Design review of the part built by this model. Coordinates are the model's own, in mm. A direction names the side the tool comes from. Give positions to 0.01 mm unless a question says otherwise; leave off trailing zeros. Order: outer loops, then holes, each group sorted by start corner. A loop starts at its lowest first (then second) coordinate and runs counter-clockwise, first axis right, second up. Notation, with made-up numbers: M -4,47.25 L 44,47.25 A34 ccw 44,77.25 Z; hole C 79,0 d5. An arc over 180 degrees is marked long. Answer as a JSON object with one key per item and string values.
Autodesk Inventor part; units mm, degrees
ref_plane "YZ Plane" through (0, 0, 0) normal (1, 0, 0) x (0, 1, 0)
ref_plane "XZ Plane" through (0, 0, 0) normal (0, 1, 0) x (-1, 0, 0)
ref_plane "XY Plane" through (0, 0, 0) normal (0, 0, 1) x (1, 0, 0)
sketch "Sketch1" plane through (0, 0, 0) normal (0, 1, 0) x (-1, 0, 0)
  line L0 (0, 0) -> (-361.95, 0)
  line L1 (-361.95, 0) -> (-361.95, -463.55)
  line L2 (-361.95, -463.55) -> (0, -463.55)
  line L3 (0, -463.55) -> (0, 0)
  dimension "d0" = 361.95
  dimension "d1" = 463.55
extrude "Extrusion1" add sketch "Sketch1" along normal blind 2.794
fillet "Fillet1" radius 19.05 4 edges at (361.95, 1.397, 0) (361.95, 1.397, -463.55) (0, 1.397, -463.55) (0, 1.397, 0)
sketch "Sketch2" plane through (0, 0, 0) normal (0, -1, 0) x (1, 0, 0)
  line L0 (19.05, 0) -> (342.9, 0)
  line L1 (342.9, 0) -> (342.9, -2.8525)
  line L2 (342.9, -2.8525) -> (19.05, -2.8525)
  line L3 (19.05, -2.8525) -> (19.05, 0)
  line L4 (342.9, -2.8525) -> (317.5, -2.8525)
  line L5 (317.5, -2.8525) -> (317.5, 0)
  line L6 (317.5, 0) -> (342.9, 0)
  line L7 (342.9, 0) -> (342.9, -2.8525)
  line L8 (19.05, -2.8525) -> (44.45, -2.8525)
  line L9 (44.45, -2.8525) -> (44.45, 0)
  line L10 (44.45, 0) -> (19.05, 0)
  line L11 (19.05, 0) -> (19.05, -2.8525)
  line L12 (44.45, -2.8525) -> (317.5, -2.8525)
  line L13 (317.5, -2.8525) -> (317.5, 0)
  line L14 (317.5, 0) -> (44.45, 0)
  line L15 (44.45, 0) -> (44.45, -2.8525)
  point P0 (0, 0)
  dimension "d5" = 25.4
  dimension "d6" = 25.4
extrude "Extrusion2" add sketch "Sketch2" along normal blind 25.4 contours L0 L5 L2 L9
sketch "Sketch3" plane through (19.05, 2.794, 0) normal (0, 0, 1) x (1, 0, 0)
  line L0 (323.85, -2.794) -> (0, -2.794)
  line L1 (25.405, -2.794) -> (25.4, -15.494)
  line L2 (25.4, -2.794) -> (25.4, -28.194)
  line L3 (25.4, -15.494) -> (85.4, -15.5178)
  line L4 (298.45, -2.794) -> (298.45, -28.194)
  line L5 (298.45, -15.494) -> (238.45, -15.494)
  circle A0 centre (85.4, -15.5178) radius 3.429
  circle A1 centre (238.45, -15.494) radius 3.429
  point P0 (-19.05, -2.794)
  dimension "d9" = 12.7
  dimension "d10" = 60
  dimension "d11" = 60
  dimension "d12" = 6.858
  dimension "d13" = 6.858
extrude "Extrusion3" cut sketch "Sketch3" against normal blind 25.4 contours A0 | A1
sketch "Sketch4" plane through (0, 2.794, 0) normal (0, 1, 0) x (1, 0, 0)
  arc A0 (0, 19.05) -> (19.05, 0) centre (19.05, 19.05) ccw
  line L0 (19.05, 0) -> (342.9, 0)
  arc A1 (342.9, 0) -> (361.95, 19.05) centre (342.9, 19.05) ccw
  line L1 (361.95, 19.05) -> (361.95, 444.5)
  arc A2 (361.95, 444.5) -> (342.9, 463.55) centre (342.9, 444.5) ccw
  line L2 (342.9, 463.55) -> (19.05, 463.55)
  arc A3 (19.05, 463.55) -> (0, 444.5) centre (19.05, 444.5) ccw
  line L3 (0, 444.5) -> (0, 19.05)
  point P0 (0, 0)
sketch "Sketch5" plane through (0, 2.794, 0) normal (0, 1, 0) x (1, 0, 0)
  arc A0 (0, 19.05) -> (19.05, 0) centre (19.05, 19.05) ccw
  line L0 (19.05, 0) -> (342.9, 0)
  arc A1 (342.9, 0) -> (361.95, 19.05) centre (342.9, 19.05) ccw
  line L1 (361.95, 19.05) -> (361.95, 444.5)
  arc A2 (361.95, 444.5) -> (342.9, 463.55) centre (342.9, 444.5) ccw
  line L2 (342.9, 463.55) -> (19.05, 463.55)
  arc A3 (19.05, 463.55) -> (0, 444.5) centre (19.05, 444.5) ccw
  line L3 (0, 444.5) -> (0, 19.05)
  line L4 (342.9, 444.5) -> (19.05, 19.05)
  line L5 (342.9, 19.05) -> (19.05, 444.5)
  line L6 (298.45, 425.45) -> (63.5, 425.45)
  line L7 (63.5, 425.45) -> (63.5, 38.1)
  line L8 (63.5, 38.1) -> (298.45, 38.1)
  line L9 (298.45, 38.1) -> (298.45, 425.45)
  line L10 (298.45, 425.45) -> (63.5, 38.1) construction
  line L11 (63.5, 425.45) -> (298.45, 38.1) construction
  point P0 (0, 0)
  point P1 (180.975, 231.775)
  dimension "d16" = 234.95
  dimension "d17" = 387.35
extrude "Extrusion4" cut sketch "Sketch5" against normal blind 25.4 contours L9 L5 L4 | L4 L5 L7 L6 L9 | L5 L9 L8 L7 L4 | L4 L7 L5
properties part number "Cart_TOP_SHELF" material "Cart Material"
(1) We need section C-C (y = -5). Write out the cut boundary in (x, z).
Checked values:
{"outline": "M 44.45,-2.85 L 317.5,-2.85 L 317.5,0 L 44.45,0 Z"}
(2) We need section A-A (z = -154). Write out the cut boundary in (x, y).
Checked values:
{"outline": "M 0,0 L 63.5,0 L 63.5,2.79 L 0,2.79 Z; M 298.45,0 L 361.95,0 L 361.95,2.79 L 298.45,2.79 Z"}
(3) Insertion check: pin 1 (0.9 mm diameter, centred on y = -19, z = -1.5, fed in from +X); pin 2 (2 mm diameter, centred on x = 287.5, y = -12, fed in from -Z); pin 3 (0.9 mm diameter, centred on y = -10, z = -1, fed in from -X). Each pin has a flat end and moves straight along its axis. Give the tip position at first contact, or say it passes through.
Checked values:
{"pin 1": "stops at x = 317.5", "pin 2": "stops at z = -2.85", "pin 3": "stops at x = 44.45"}
(4) Tool access review of faces 1 (the cylindrical face through (5.43, 1.42, -5.73)), 2 (the flat face through (183, -13, -2.852)): name each direction out of +Z, -Z, +X, -X, +Y, -Y from which nothing blocks a thin tool from reaching the whole face with its end or side.
Checked values:
{"face 1": "+Z, -X, +Y, -Y", "face 2": "-Z, +X, -X, -Y"}
(5) To check wall thickness, follow L1, parallel to Y at x = 104.45, z = -0.9; L2, parallel to Y at x = 257, z = -1; L3, parallel to Y at x = 38, z = -264. State the ranges of each line that lie inside material, in increasing order. Write a range as from..to.
Checked values:
{"L1": "y = -25.4..-16.15, -9.29..2.79", "L2": "y = -25.4..-16.09, -9.31..2.79", "L3": "y = 0..2.79"}
(6) We need section B-B (x = 244). Write out the cut boundary in (y, z).
Checked values:
{"outline": "M -25.4,-2.85 L 0,-2.85 L 0,-38.1 L 2.79,-38.1 L 2.79,0 L -25.4,0 Z; M 0,-463.55 L 2.79,-463.55 L 2.79,-425.45 L 0,-425.45 Z"}
